Part model, mm, in its own coordinate system. Give positions to 0.01 mm unless a question says otherwise; leave off trailing zeros. Write each loop counter-clockwise with the first axis right and the second up, starting at its lowest first coordinate (ties: lowest second). Pieces come first, ordered by that corner, then holes. Notation, with made-up numbers: M -23,48 L 18,48 A19 ccw 18,52 Z; hole C -31,37 d1. An arc over 180 degrees is marked long. Use a Markdown table: item, result.
Autodesk Inventor part; units mm, degrees
ref_plane "YZ Plane" through (0, 0, 0) normal (1, 0, 0) x (0, 1, 0)
ref_plane "XZ Plane" through (0, 0, 0) normal (0, 1, 0) x (-1, 0, 0)
ref_plane "XY Plane" through (0, 0, 0) normal (0, 0, 1) x (1, 0, 0)
sketch "Sketch1" plane through (0, 0, 0) normal (0, 0, 1) x (1, 0, 0)
  line L0 (-12.1708, 16.0073) -> (13.2292, 16.0073)
  line L1 (13.2292, 16.0073) -> (13.2292, -34.7927)
  line L2 (13.2292, -34.7927) -> (-12.1708, -34.7927)
  line L3 (-12.1708, -34.7927) -> (-12.1708, 16.0073)
  line L4 (11.9592, 14.7373) -> (-10.9008, 14.7373)
  line L5 (-10.9008, 14.7373) -> (-10.9008, -33.5227)
  line L6 (-10.9008, -33.5227) -> (11.9592, -33.5227)
  line L7 (11.9592, -33.5227) -> (11.9592, 14.7373)
  point P0 (0, 0)
  dimension "d0" = 25.4
  dimension "d1" = 50.8
  dimension "d2" = 1.27
extrude "Extrusion1" add sketch "Sketch1" along normal blind 711.2
sketch "Sketch2" plane through (-12.1708, 16.0073, 0) normal (0, 1, 0) x (1, 0, 0)
  circle A0 centre (12.7, -12.7) radius 1.7272
  line L0 (25.4, 0) -> (0, 0)
  line L1 (0, 0) -> (0, -711.2)
  point P0 (12.1708, 0)
  dimension "d5" = 3.4544
  dimension "d6" = 12.7
  dimension "d7" = 12.7
extrude "Extrusion2" cut sketch "Sketch2" against normal through all
pattern_linear "Rectangular Pattern1" count 71 spacing 25.4 along (0, 0, 1) of "Extrusion2"
sketch "Sketch3" plane through (13.2292, -34.7927, 0) normal (1, 0, 0) x (0, 0, -1)
  circle A0 centre (-101.6, 25.4) radius 19.05
  circle A1 centre (-101.6, 25.4) radius 23.8125 construction
  circle A2 centre (-125.4125, 25.4) radius 2.4892
  circle A3 centre (-77.7875, 25.4) radius 2.4892
  line L0 (-406.4, 34.925) -> (-381, 15.875) construction
  line L1 (-711.2, 50.8) -> (-711.2, 0) construction
  line L2 (-711.2, 25.4) -> (0, 25.4) construction
  line L3 (0, 50.8) -> (0, 0) construction
  circle A4 centre (-609.6, 25.4) radius 14.2875
  circle A5 centre (-355.6, 25.4) radius 14.2875
  circle A6 centre (-44.45, 25.4) radius 6.35
  circle A7 centre (-158.75, 25.4) radius 6.35
  line L4 (0, 0) -> (0, 50.8)
  point P0 (0, 34.7927)
  point P1 (-393.7, 25.4)
  point P2 (-624.3413, 25.4)
  point P3 (-134.62, 25.4)
  dimension "d15" = 38.1
  dimension "d16" = 47.625
  dimension "d17" = 4.9784
  dimension "d18" = 4.9784
  dimension "d25" = 28.575
  dimension "d27" = 28.575
  dimension "d29" = 12.7
  dimension "d30" = 12.7
  dimension "d31" = 355.6
  dimension "d33" = 101.6
  dimension "d34" = 101.6
  dimension "d35" = 57.15
  dimension "d36" = 57.15
  dimension "d37" = 77.7875
  dimension "d38" = 125.4125
  dimension "d39" = 158.75
  dimension "d40" = 44.45
extrude "Extrusion3" cut sketch "Sketch3" against normal through all
equation "\"d3\" = d13"
equation "\"d31\" = 0.5 * d13"
equation "\"d33\" = d32"
equation "\"d34\" = d32"
equation "\"d10\" = d14"
equation "\"d13\" = 711.2"
equation "\"d14\" = d13"
equation "\"d32\" = 101.6"
properties part number "VersaFrame 28in"
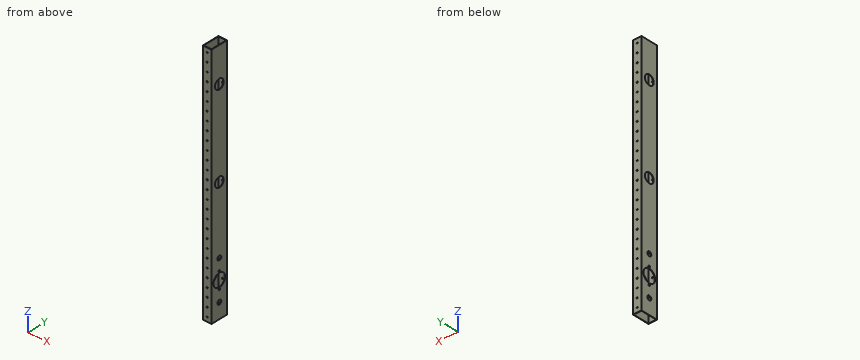
1. Cut at B-B, the plane z = 356.5. Give the cut face in (x, y), then the cut area to 3 significant figures.
Findings below:
| item | result |
|---|---|
| outline | M -12.17,-34.79 L 13.23,-34.79 L 13.23,-23.65 L 11.96,-23.65 L 11.96,-33.52 L -10.9,-33.52 L -10.9,-23.65 L -12.17,-23.65 Z; M -12.17,4.87 L -10.9,4.87 L -10.9,14.74 L 11.96,14.74 L 11.96,4.87 L 13.23,4.87 L 13.23,16.01 L -12.17,16.01 Z |
| area | 115 mm2 |
2. Drill centre lines: L1, parallel to Y at x = -3.5, z = 72.5; L2, parallel to X at y = -3, z = 646; L3, parallel to Y at x = -11.4, z = 355.6. Where is each one in solid material? Low to high.
Findings below:
| item | result |
|---|---|
| L1 | -34.79 to -33.52, 14.74 to 16.01 |
| L2 | -12.17 to -10.9, 11.96 to 13.23 |
| L3 | -34.79 to -23.68, 4.89 to 16.01 |
3. Cut at A-A, the plane z = 175. Give the cut face in (x, y), then the cut area to 3 significant figures.
Findings below:
| item | result |
|---|---|
| outline | M -12.17,-34.79 L 13.23,-34.79 L 13.23,16.01 L -12.17,16.01 Z; hole M -10.9,-33.52 L 11.96,-33.52 L 11.96,14.74 L -10.9,14.74 Z |
| area | 187 mm2 |
